```python
from build123d import *

# Parameters (mm, degrees)
SKETCH_1_R          = 1.55
EXTRUDE_1_DEPTH     = 3
FILLET_1_R          = 1.1
SKETCH_2_W          = 5.927431674
SKETCH_2_H          = 6.747498384
CUT_EXTRUDE_1_DEPTH = 10
FILLET_2_R          = 2


with BuildPart() as part:
    # 草图1 → 凸台-拉伸1 (new body)
    with BuildSketch(Plane(origin=(0, 0, 0), x_dir=(0, 0, -1), z_dir=(1, 0, 0))):
        with BuildLine():
            ThreePointArc((-42, -68.5), (-40.95, -67.45), (-39.9, -68.5))
            Line((-39.9, -68.5), (-39.9, -71.6))
            Line((-39.9, -71.6), (-31.9, -71.6))
            Line((-31.9, -71.6), (-31.9, -68.5))
            ThreePointArc((-31.9, -68.5), (-30.85, -67.45), (-29.8, -68.5))
            Line((-29.8, -68.5), (-26.9, -68.5))
            ThreePointArc((-26.9, -68.5), (-21.67999009, -41.785074582), (-6.787840486, -19))
            Line((-6.787840486, -19), (7.5, -19))
            Line((7.5, -19), (7.5, 4))
            Line((7.5, 4), (-7.5, 4))
            ThreePointArc((-7.5, 4), (-34.999100763, -27.710877676), (-44.9, -68.5))
            Line((-44.9, -68.5), (-42, -68.5))
        make_face()
        with BuildLine():
            Line((-30.793215628, -64.5), (-40.805797705, -64.5))
            ThreePointArc((-40.805797705, -64.5), (-40.271828479, -58.18700937), (-39.268965575, -51.931352743))
            Line((-39.268965575, -51.931352743), (-29.460918095, -53.881277009))
            ThreePointArc((-29.460918095, -53.881277009), (-30.316784958, -59.166835176), (-30.793215628, -64.5))
        make_face(mode=Mode.SUBTRACT)
        with BuildLine():
            Line((-34.979756463, -37.338397808), (-25.805292651, -41.334732969))
            ThreePointArc((-25.805292651, -41.334732969), (-27.472904513, -46.09199558), (-28.817045963, -50.950571569))
            Line((-28.817045963, -50.950571569), (-38.539210298, -48.609733975))
            ThreePointArc((-38.539210298, -48.609733975), (-36.955711073, -42.91209778), (-34.979756463, -37.338397808))
        make_face(mode=Mode.SUBTRACT)
        with BuildLine():
            Line((-28.576156327, -24.426712573), (-20.026519864, -29.613591821))
            ThreePointArc((-20.026519864, -29.613591821), (-22.494886937, -34.009003163), (-24.662290725, -38.560358752))
            Line((-24.662290725, -38.560358752), (-33.830271356, -34.566847621))
            ThreePointArc((-33.830271356, -34.566847621), (-31.373767539, -29.408407631), (-28.576156327, -24.426712573))
        make_face(mode=Mode.SUBTRACT)
        with BuildLine():
            Line((-19.554533637, -12.18081642), (-12.300184819, -19.073994509))
            ThreePointArc((-12.300184819, -19.073994509), (-15.49430702, -22.974002232), (-18.419117678, -27.079846784))
            Line((-18.419117678, -27.079846784), (-26.754350152, -21.555002932))
            ThreePointArc((-26.754350152, -21.555002932), (-23.317641268, -16.742564875), (-19.554533637, -12.18081642))
        make_face(mode=Mode.SUBTRACT)
        with Locations((0, -15)):
            Circle(SKETCH_1_R, mode=Mode.SUBTRACT)
        with BuildLine():
            ThreePointArc((-17.526444973, -9.969558223), (-12.691914425, -5.270049035), (-7.5, -0.968642657))
            Line((-7.5, -0.968642657), (-7.5, -14.084287323))
            ThreePointArc((-7.5, -14.084287323), (-8.906765299, -15.452898351), (-10.277222475, -16.857865213))
            Line((-10.277222475, -16.857865213), (-17.526444973, -9.969558223))
        make_face(mode=Mode.SUBTRACT)
        Circle(SKETCH_1_R, mode=Mode.SUBTRACT)
    extrude(amount=EXTRUDE_1_DEPTH)

    # 圆角1
    fillet_1_edges = [part.edges().sort_by_distance(p)[0] for p in [
        (1.5, -12.18081642, 19.554533637),
        (1.5, -21.555002932, 26.754350152),
        (1.5, -27.079846784, 18.419117678),
        (1.5, -19.073994509, 12.300184819),
        (1.5, -24.426712573, 28.576156327),
        (1.5, -34.566847621, 33.830271356),
        (1.5, -38.560358752, 24.662290725),
        (1.5, -29.613591821, 20.026519864),
        (1.5, -51.931352743, 39.268965575),
        (1.5, -64.5, 40.805797705),
        (1.5, -64.5, 30.793215628),
        (1.5, -53.881277009, 29.460918095),
        (1.5, -37.338397808, 34.979756463),
        (1.5, -48.609733975, 38.539210298),
        (1.5, -50.950571569, 28.817045963),
        (1.5, -41.334732969, 25.805292651),
        (1.5, -0.968642657, 7.5),
        (1.5, -9.969558223, 17.526444973),
        (1.5, -16.857865213, 10.277222475),
        (1.5, -14.084287323, 7.5),
    ]]
    fillet(fillet_1_edges, radius=FILLET_1_R)

    # 草图2 → 切除-拉伸1 (cut)
    with BuildSketch(Plane(origin=(3, 0, 0), x_dir=(0, 0, -1), z_dir=(1, 0, 0))):
        with Locations((-15.463715837, 0.173749192)):
            Rectangle(SKETCH_2_W, SKETCH_2_H)
    extrude(amount=-CUT_EXTRUDE_1_DEPTH, mode=Mode.SUBTRACT)

    # 圆角2
    fillet_2_edges = [part.edges().sort_by_distance(p)[0] for p in [
        (1.5, 0.16980982, 12.5),
        (1.5, -3.2, 16.358570309),
        (1.5, -3.2, 12.5),
        (1.5, 4, 7.5),
    ]]
    fillet(fillet_2_edges, radius=FILLET_2_R)


solid = part.part
```
Check sheet for the modelled part. Datum: model origin and axes. Units: mm. A direction names the side the tool comes from. Give positions to 0.01 mm unless a question says otherwise; leave off trailing zeros. Order: outer loops, then holes, each group sorted by start corner. A loop starts at its lowest first (then second) coordinate and runs counter-clockwise, first axis right, second up. Notation, with made-up numbers: M -22,-4.75 L -5,-4.75 A32 ccw -5,24.25 Z; hole C 25.5,-2 d5. An arc over 180 degrees is marked long. Answer in a Markdown table with one row per item. Add a question column.
Q1. Thickness scan on L1, parallel to Y at x = 1.65, z = 0; L2, parallel to Y at x = 0.55, z = 21; L3, parallel to Z at x = 2.05, y = -68. Record the ranges inside material, lowest first.
Q2. Sectioned sample at C-C, the plane x = 2.05. Count the separate pieces of the cut face and the enclosed holes in it, and give its area (3 significant figures).
Q3. Gauge pin test, flat ends, axial feed: pin 1 Ø3 at (y, z) = (-15, 0) entering from +X; pin 2 Ø0.9 at (x, y) = (2, -70) entering from +Z; pin 3 Ø1 at (x, y) = (1.5, -10) entering from +Z; pin 4 Ø0.5 at (x, y) = (1.5, -1) entering from +Z. Record the tip position at first contact, or that the pin passes through.
Q4. Sectioned sample at D-D, the plane y = 0. Record the boundary of the cut face in (x, z), and give its area (3 significant figures).
Q5. Release check for a two-part mould opening along Y. For faces 1 (the cylindrical face through (1.48, -32.77, 37.41)), 2 (the cylindrical face through (1.48, -67.45, 40.97)), 3 (the cylindrical face through (1.52, -26.64, 18.52)) record: released by +Y, released by -Y, zero draft, split by the parting line, or undercut.
Q6. Access from +Z, -Z, +X, -X, +Y, -Y to the whole of each face (thin tool, end or side, straight path). Record for faces 4 (the flat face through (1, -71.6, 36)), 5 (the cylindrical face through (1.479, -42.995, 36.982)).
Q7. Sectioned sample at B-B, the plane y = -62.5. Record the boundary of the cut face in (x, z), and give its area (3 significant figures).
Q8. Sectioned sample at A-A, the plane z = 0. Record the boundary of the cut face in (x, y).
Verdict:
| question | item | result |
|---|---|---|
| 1 | L1 | -19 to -16.55, -13.45 to -1.55, 1.55 to 4 |
| 1 | L2 | -40.17 to -31.27, -29.02 to -25.37, -13.86 to -7.82 |
| 1 | L3 | 26.9 to 29.93, 31.77 to 40.03, 41.87 to 44.9 |
| 2 | separate pieces | 1 |
| 2 | enclosed holes | 7 |
| 2 | area | 1,070 mm² |
| 3 | pin 1 | through |
| 3 | pin 2 | z = 39.9 |
| 3 | pin 3 | z = 23.4 |
| 3 | pin 4 | z = 12.5 |
| 4 | outline | M 0,-7.5 L 3,-7.5 L 3,-1.55 L 0,-1.55 Z; M 0,1.55 L 3,1.55 L 3,12.34 L 0,12.34 Z |
| 4 | area | 50.2 mm² |
| 5 | face 1 | released by +Y |
| 5 | face 2 | released by -Y |
| 5 | face 3 | undercut |
| 6 | face 4 | +Z, -Z, +X, -X, -Y |
| 6 | face 5 | +X, -X |
| 7 | outline | M 0,26.65 L 3,26.65 L 3,30.66 L 0,30.66 Z; M 0,40.69 L 3,40.69 L 3,44.7 L 0,44.7 Z |
| 7 | area | 24.1 mm² |
| 8 | outline | M 0,-19 L 3,-19 L 3,-16.55 L 0,-16.55 Z; M 0,-13.45 L 3,-13.45 L 3,-1.55 L 0,-1.55 Z; M 0,1.55 L 3,1.55 L 3,4 L 0,4 Z |
